Check sheet for the modelled part. Datum: model origin and axes. Units: mm. A direction names the side the tool comes from. Round coordinates to 2 decimals unless told otherwise and drop trailing zeros. Loops run counter-clockwise (first coordinate to the right, second up) from the corner with the lowest first, then second, coordinate; pieces in that order, holes last. Notation, with made-up numbers: (45.5, 67.25) -> (53.5, 67.25) arc R26 cw to (53.5, 104.25) -> close; hole circle Ø8 at (27, 32.25). An arc over 180 degrees is marked (long way). Return JSON: item names as keys, results as strings.
from build123d import *

# Parameters (mm, degrees)
BOSS_EXTRUDE1_DEPTH            = 12
F_4_8_4_8_DIAMETER_HOLE1_D     = 4.8
F_4_8_4_8_DIAMETER_HOLE1_DEPTH = 8
F_4_8_4_8_DIAMETER_HOLE1_TIP   = 1.442065486
F_4_8_4_8_DIAMETER_HOLE2_D     = 4.8
F_4_8_4_8_DIAMETER_HOLE2_DEPTH = 8
F_4_8_4_8_DIAMETER_HOLE2_TIP   = 1.442065486
CUT_EXTRUDE1_REACH             = 104.772
SKETCH11_W                     = 9
SKETCH11_H                     = 14
FILLET1_R                      = 1


with BuildPart() as part:
    # Sketch1 → Boss-Extrude1 (new, symmetric)
    with BuildSketch(Plane.XY):
        Polygon((0, 0), (-23, 0), (-31, 0), (-31, 77), (-23.404895261, 77), (36, 77), (36, 41), (27, 41), (27, 69), (-23, 69), (-23, 27.5), (0, 27.5), align=None)
    extrude(amount=BOSS_EXTRUDE1_DEPTH, both=True)

    # Ø4.8 (4.8) Diameter Hole1
    with Locations(Plane(origin=(0, 41, 0), x_dir=(-1, 0, 0), z_dir=(0, -1, 0))):
        with Locations((-31.3, 4.875), (-31.3, -4.875)):
            Hole(F_4_8_4_8_DIAMETER_HOLE1_D / 2, depth=F_4_8_4_8_DIAMETER_HOLE1_DEPTH)
            with Locations((0, 0, -(F_4_8_4_8_DIAMETER_HOLE1_DEPTH + F_4_8_4_8_DIAMETER_HOLE1_TIP / 2))):  # 118° drill point
                Cone(0, F_4_8_4_8_DIAMETER_HOLE1_D / 2, F_4_8_4_8_DIAMETER_HOLE1_TIP, mode=Mode.SUBTRACT)

    # Ø4.8 (4.8) Diameter Hole2
    with Locations(Plane(origin=(0, 0, 0), x_dir=(-1, 0, 0), z_dir=(0, -1, 0))):
        with Locations((5.95, 0), (21.95, 0)):
            Hole(F_4_8_4_8_DIAMETER_HOLE2_D / 2, depth=F_4_8_4_8_DIAMETER_HOLE2_DEPTH)
            with Locations((0, 0, -(F_4_8_4_8_DIAMETER_HOLE2_DEPTH + F_4_8_4_8_DIAMETER_HOLE2_TIP / 2))):  # 118° drill point
                Cone(0, F_4_8_4_8_DIAMETER_HOLE2_D / 2, F_4_8_4_8_DIAMETER_HOLE2_TIP, mode=Mode.SUBTRACT)

    # Sketch11 → Cut-Extrude1 (cut, up to next)
    with BuildSketch(Plane(origin=(36, 0, 0), x_dir=(0, 0, -1), z_dir=(1, 0, 0)), mode=Mode.PRIVATE) as cut_extrude1_sk1:
        with Locations((0, 62)):
            Rectangle(SKETCH11_W, SKETCH11_H)
    cut_extrude1_tool1 = extrude(cut_extrude1_sk1.sketch, amount=-CUT_EXTRUDE1_REACH, mode=Mode.PRIVATE) & part.part
    add(cut_extrude1_tool1.solids().sort_by_distance((36, 62, 0))[0], mode=Mode.SUBTRACT)

    # Fillet1
    fillet1_edges = [part.edges().sort_by_distance(p)[0] for p in [
        (-15.5, 0, -12),
        (-23, 48.25, 12),
        (-31, 38.5, -12),
        (2.5, 77, -12),
        (36, 59, -12),
        (31.5, 41, -12),
        (27, 55, -12),
        (2, 69, -12),
        (-23, 48.25, -12),
        (-11.5, 27.5, -12),
        (0, 13.75, -12),
        (2, 69, 12),
        (0, 0, 0),
        (-31, 0, 0),
        (27, 55, 12),
        (-31, 77, 0),
        (36, 77, 0),
        (36, 41, 0),
        (27, 41, 0),
        (0, 27.5, 0),
        (31.5, 41, 12),
        (36, 59, 12),
        (2.5, 77, 12),
        (-31, 38.5, 12),
        (-15.5, 0, 12),
        (0, 13.75, 12),
        (36, 62, 4.5),
        (36, 55, 0),
        (36, 62, -4.5),
        (36, 69, 0),
        (27, 55, 0),
        (27, 62, 4.5),
        (27, 62, -4.5),
        (-11.5, 27.5, 12),
    ]]
    fillet(fillet1_edges, radius=FILLET1_R)


solid = part.part
Q1. Go/stop test with flat-tipped pins: pin 1 (3 mm diameter, centred on x = -5.95, z = 0, fed in from -Y); pin 2 (4.5 mm diameter, centred on x = 31.3, z = 4.875, fed in from -Y); pin 3 (8 mm diameter, centred on y = 17, z = -3.5, fed in from +X). Record where each tip stops, or that it passes through.
Results list:
{"pin 1": "y = 8.54", "pin 2": "y = 49.09", "pin 3": "x = 0"}
Q2. Section check A-A (y = 63). Record the boundary of the cut face in (x, z), then the cut area to 3 significant figures.
Results list:
{"outline": "(-31, -11) arc R1 ccw to (-30, -12) -> (-24, -12) arc R1 ccw to (-23, -11) -> (-23, 11) arc R1 ccw to (-24, 12) -> (-30, 12) arc R1 ccw to (-31, 11) -> close; (27, -11) arc R1 ccw to (28, -12) -> (35, -12) arc R1 ccw to (36, -11) -> (36, -5.5) arc R1 ccw to (35, -4.5) -> (28, -4.5) arc R1 ccw to (27, -5.5) -> close; (27, 5.5) arc R1 ccw to (28, 4.5) -> (35, 4.5) arc R1 ccw to (36, 5.5) -> (36, 11) arc R1 ccw to (35, 12) -> (28, 12) arc R1 ccw to (27, 11) -> close", "area": "324 mm^2"}
Q3. Draft check along Z on faces 5 (the flat face through (-7, 25, 12)), 6 (the conical face through (31.7, 50.2, -4.9)), 7 (the flat face through (32, 41, 0)). Enter one of: released by +Z, released by -Z, zero draft, split by the parting line, or undercut.
Results list:
{"face 5": "released by +Z", "face 6": "undercut", "face 7": "zero draft"}
Q4. Section check C-C (z = 10). Record the boundary of the cut face in (x, y), then the cut area to 3 significant figures.
Results list:
{"outline": "(-31, 1) arc R1 ccw to (-30, 0) -> (-1, 0) arc R1 ccw to (0, 1) -> (0, 26.5) arc R1 ccw to (-1, 27.5) -> (-23, 27.5) -> (-23, 69) -> (27, 69) -> (27, 42) arc R1 ccw to (28, 41) -> (35, 41) arc R1 ccw to (36, 42) -> (36, 76) arc R1 ccw to (35, 77) -> (-30, 77) arc R1 ccw to (-31, 76) -> close", "area": "1,970 mm^2"}
Q5. Tool access check on faces 1 (the flat face through (-23, 49, 0)), 2 (the cylindrical face through (-24.348, 4.056, -0.106)), 3 (the flat face through (32, 55, 0)), 4 (the flat face through (27, 52, 0)). Record the directions out of +Z, -Z, +X, -X, +Y, -Y that give a thin tool (end or side, any length) a straight path to the whole face; none if there is none.
Results list:
{"face 1": "+Z, -Z", "face 2": "-Y", "face 3": "+X", "face 4": "+Z, -Z, -Y"}
Q6. Material ranges on line 1 (X direction, y = 46, z = -5); line 2 (Z direction, x = 31.3, y = 46.25) (3 decimals); line 3 (Y direction, x = -2, z = -3.75), recorded low to high.
Results list:
{"line 1": "-31 to -23, 27 to 28.9, 33.7 to 36", "line 2": "-12 to -7.275, -2.475 to 2.475, 7.275 to 12", "line 3": "0 to 27.5, 69 to 77"}
Q7. Section check D-D (y = 19). Record the boundary of the cut face in (x, z).
Results list:
{"outline": "(-31, -11) arc R1 ccw to (-30, -12) -> (-1, -12) arc R1 ccw to (0, -11) -> (0, 11) arc R1 ccw to (-1, 12) -> (-30, 12) arc R1 ccw to (-31, 11) -> close"}
Q8. Section check B-B (x = -17). Record the boundary of the cut face in (y, z), then the cut area to 3 significant figures.
Results list:
{"outline": "(0, -11) arc R1 ccw to (1, -12) -> (26.5, -12) arc R1 ccw to (27.5, -11) -> (27.5, 11) arc R1 ccw to (26.5, 12) -> (1, 12) arc R1 ccw to (0, 11) -> close; (69, -11) arc R1 ccw to (70, -12) -> (76, -12) arc R1 ccw to (77, -11) -> (77, 11) arc R1 ccw to (76, 12) -> (70, 12) arc R1 ccw to (69, 11) -> close", "area": "850 mm^2"}
